```python
from build123d import *

# Parameters (mm, degrees)
F0_R     = 3.75
F1_DEPTH = 18
F3_DEPTH = 13
F4_R     = 1.3
F5_DEPTH = 18.001


with BuildPart() as f1:
    # F0 (on Front) → F1 (new body)
    with BuildSketch(Plane.XZ):
        Circle(F0_R)
    extrude(amount=F1_DEPTH)

    # F2 (on face) → F3 (cut, through all)
    with BuildSketch(Plane(origin=(0, 0, 0), x_dir=(-1, 0, 0), z_dir=(0, 1, 0))):
        with BuildLine():
            Line((2.4, -1.6278820596), (2.4, 1.6278820596))
            ThreePointArc((2.4, 1.6278820596), (-2.9, 0), (2.4, -1.6278820596))
        make_face()
    extrude(amount=-F3_DEPTH, mode=Mode.SUBTRACT)

    # F4 (on face) → F5 (cut, through all)
    with BuildSketch(Plane.XZ.offset(18)):
        Circle(F4_R)
    extrude(amount=-F5_DEPTH, mode=Mode.SUBTRACT)


solid = f1.part
```
For this review, take the finished solid that the model builds, in its own axes (mm). A direction names the side the tool comes from. Coordinates: 2 decimals unless noted, no trailing zeros. Order: outer loops, then holes, each group sorted by start corner. A loop starts at its lowest first (then second) coordinate and runs counter-clockwise, first axis right, second up. Notation, with made-up numbers: (-19, -5.5) - (1, -5.5) arc R26 ccw to (1, 24.5) - close; hole circle Ø7 at (-18.5, -5.75). An arc over 180 degrees is marked (long way). Answer as a JSON object with one key per item and string values. Group by question number.
1. We need section D-D on z = 2.5. State the section outline as (x, y) points, then the cut area to 3 significant figures.
2. We need section A-A on x = 0. State the section outline as (y, z) points, then the cut area to 3 significant figures.
3. We need section B-B on z = 0. State the section outline as (x, y) points.
4. For probe 1 along Z at (x, y) = (0, -3.5); probe 2 along Z at (x, y) = (0, -15.55); probe 3 along Y at (x, z) = (-0.5, 1.75), list the stretches that pass through material, from the lowest coordinate up.
5. For faces 4 (the cylindrical face through (2.9, -6.4, 0.1)), 5 (the flat face through (2, -18, 0)), list the 3-axis set-ups (+Z, -Z, +X, -X, +Y, -Y) from which the entire face can be reached by the end or side of a thin tool; tool diameter is ignored.
6. The part is to be moulded in two halves that separate along Z. For faces 1 (the flat face through (-3, 0, 0)), 2 (the cylindrical face through (-3.746, -8.874, 0.165)), 3 (the flat face through (1.5, -13, 0)), say which applies: pulls with the +Z half, pulls with the -Z half, needs draft (parallel to the pull), parting line crosses it, or undercut.
7. We need section C-C on y = -11.5. State the section outline as (x, z) points, then the cut area to 3 significant figures.
8. Clearance check with flat-ended pins moving along their axes: P1, Ø4, axis at y = -5.5, z = -2.5, coming from the -X side; P2, Ø2.5, axis at x = 0, z = 1, coming from the +Y side; P3, Ø2.5, axis at x = 0, z = 0, coming from the +Y side; P4, Ø2, axis at y = -4, z = -2, coming from the -X side. State where each tip first meets the part, or that it passes through.
Final values:
{
 "1": {"outline": "(-2.8, -18) - (2.8, -18) - (2.8, 0) - (1.47, 0) - (1.47, -13) - (-1.47, -13) - (-1.47, 0) - (-2.8, 0) - close", "area": "62.4 mm²"},
 "2": {"outline": "(-18, -3.75) - (0, -3.75) - (0, -2.9) - (-13, -2.9) - (-13, -1.3) - (-18, -1.3) - close; (-18, 1.3) - (-13, 1.3) - (-13, 2.9) - (0, 2.9) - (0, 3.75) - (-18, 3.75) - close", "area": "46.6 mm²"},
 "3": {"outline": "(-3.75, -18) - (-1.3, -18) - (-1.3, -13) - (-2.4, -13) - (-2.4, 0) - (-3.75, 0) - close; (1.3, -18) - (3.75, -18) - (3.75, 0) - (2.9, 0) - (2.9, -13) - (1.3, -13) - close"},
 "4": {"probe 1": "-3.75 to -2.9, 2.9 to 3.75", "probe 2": "-3.75 to -1.3, 1.3 to 3.75", "probe 3": "-18 to -13"},
 "5": {"face 4": "+Y", "face 5": "+Z, -Z, +X, -X, -Y"},
 "6": {"face 1": "needs draft", "face 2": "parting line crosses it", "face 3": "undercut"},
 "7": {"outline": "circle Ø7.5 at (0, 0); hole (-2.4, -1.63) arc R2.9 ccw (long way) to (-2.4, 1.63) - close", "area": "18.9 mm²"},
 "8": {"P1": "x = -3.72", "P2": "y = -13", "P3": "through", "P4": "x = -3.61"}
}
